Input: part model. Units: mm. Frame: model coordinates. A direction names the side the tool comes from. Round coordinates to 2 decimals unless told otherwise and drop trailing zeros. Loops run counter-clockwise (first coordinate to the right, second up) from the corner with the lowest first, then second, coordinate; pieces in that order, holes last. Notation, with made-up numbers: (-29.75, 12.25) -> (-18.75, 12.25) arc R29 ccw to (-18.75, 40.25) -> close; hole circle Ø5 at (-20, 30.25). An arc over 180 degrees is marked (long way). Answer in a Markdown table with one row per item. Add a question column.
Q1. Mould query, pull axis X, two halves, no side actions, for faces 5 (the face through (-103.049, 3, -23)), 6 (the face through (-40, 3, 61.274)), 7 (the face through (-148, 3, 116.519)), 8 (the face through (-128.449, 3, -23)). Classes: pulls with the +X half, pulls with the -X half, needs draft (parallel to the pull), parting line crosses it, or undercut.
Q2. Pin query (flat end, axial travel): pin 1 (1 mm diameter, centred on x = 1.5, y = 3, fed in from +Z); pin 2 (3.5 mm diameter, centred on y = 2, z = 73.5, fed in from +X); pin 3 (1.4 mm diameter, centred on x = 68.5, y = 4.5, fed in from -Z). Return the tip coordinate at first contact, or that it passes through.
Q3. Ray query, L1, parallel to X at y = 2.75, z = -17; L2, parallel to X at y = 5.5, z = 25; L3, parallel to X at y = 0.5, z = 34.5. Return the intervals inside material, ascending. Write a range as from..to.
Q4. Section B-B, the plane x = 21.5. Output: boundary loops of the cut face in (y, z), and give its area (3 significant figures).
Q5. Section C-C, the plane y = 4.5. Give the number of separate pieces and of enclosed holes in the cut face, and give its area (3 significant figures).
Q6. Reachability of faces 1 (the face through (49, 3, 19.999)), 2 (the face through (-128.449, 3, 120)), 3 (the face through (-103.049, 3, 120)), 4 (the face through (78, 3, 35.874)) from +Z, -Z, +X, -X, +Y, -Y: full face, straight path, thin tool, end or side. Return the list, or none.
Q7. Section A-A, the plane x = 50. Output: boundary loops of the cut face in (y, z), and give its area (3 significant figures).
```python
from build123d import *

# Parameters (mm, degrees)
SKETCH1_R           = 1.5875
SKETCH1_W           = 6.35
SKETCH1_H           = 25.4
BOSS_EXTRUDE1_DEPTH = 6.35


with BuildPart() as part:
    # Sketch1 → Boss-Extrude1 (new body)
    with BuildSketch(Plane(origin=(0, 0, 0), x_dir=(1, 0, 0), z_dir=(0, 1, 0))):
        Polygon((-153.849110766, 19.370876928), (-153.849110766, -116.519123072), (-142.673040444, -116.519123072), (-142.673040444, -113.344123072), (-144.425640444, -113.344123072), (-144.425640444, -110.804123072), (-142.673040444, -110.804123072), (-142.673040444, -109.534123072), (-139.625181088, -109.534123072), (-139.625181088, -110.804123072), (-137.872581088, -110.804123072), (-137.872581088, -113.344123072), (-139.625181088, -113.344123072), (-139.625181088, -116.519123072), (-128.449110766, -116.519123072), (-128.449110766, -122.869123072), (-103.049110766, -122.869123072), (-103.049110766, -116.519123072), (-91.873040444, -116.519123072), (-91.873040444, -113.344123072), (-93.625640444, -113.344123072), (-93.625640444, -110.804123072), (-91.873040444, -110.804123072), (-91.873040444, -109.534123072), (-88.825181088, -109.534123072), (-88.825181088, -110.804123072), (-87.072581088, -110.804123072), (-87.072581088, -113.344123072), (-88.825181088, -113.344123072), (-88.825181088, -116.519123072), (-77.649110766, -116.519123072), (74.750889234, -116.519123072), (81.100889234, -116.519123072), (81.100889234, -86.674123072), (74.750889234, -86.674123072), (74.750889234, -75.49805275), (71.575889234, -75.49805275), (71.575889234, -77.25065275), (69.035889234, -77.25065275), (69.035889234, -75.49805275), (67.765889234, -75.49805275), (67.765889234, -72.450193394), (69.035889234, -72.450193394), (69.035889234, -70.697593394), (71.575889234, -70.697593394), (71.575889234, -72.450193394), (74.750889234, -72.450193394), (74.750889234, -61.274123072), (81.100889234, -61.274123072), (81.100889234, -35.874123072), (74.750889234, -35.874123072), (74.750889234, -24.69805275), (71.575889234, -24.69805275), (71.575889234, -26.45065275), (69.035889234, -26.45065275), (69.035889234, -24.69805275), (67.765889234, -24.69805275), (67.765889234, -21.650193394), (69.035889234, -21.650193394), (69.035889234, -19.897593394), (71.575889234, -19.897593394), (71.575889234, -21.650193394), (74.750889234, -21.650193394), (74.750889234, -10.474123072), (81.100889234, -10.474123072), (81.100889234, 19.370876928), (74.750889234, 19.370876928), (-77.649110766, 19.370876928), (-88.825181088, 19.370876928), (-88.825181088, 16.195876928), (-87.072581088, 16.195876928), (-87.072581088, 13.655876928), (-88.825181088, 13.655876928), (-88.825181088, 12.385876928), (-91.873040444, 12.385876928), (-91.873040444, 13.655876928), (-93.625640444, 13.655876928), (-93.625640444, 16.195876928), (-91.873040444, 16.195876928), (-91.873040444, 19.370876928), (-103.049110766, 19.370876928), (-103.049110766, 25.720876928), (-128.449110766, 25.720876928), (-128.449110766, 19.370876928), (-139.625181088, 19.370876928), (-139.625181088, 16.195876928), (-137.872581088, 16.195876928), (-137.872581088, 13.655876928), (-139.625181088, 13.655876928), (-139.625181088, 12.385876928), (-142.673040444, 12.385876928), (-142.673040444, 13.655876928), (-144.425640444, 13.655876928), (-144.425640444, 16.195876928), (-142.673040444, 16.195876928), (-142.673040444, 19.370876928), align=None)
        with Locations(Location((-39.549110766, 2.225876928, 0), (0, 0, 270))):
            Circle(SKETCH1_R, mode=Mode.SUBTRACT)
        with Locations(Location((-39.549110766, -48.574123072, 0), (0, 0, 270))):
            Circle(SKETCH1_R, mode=Mode.SUBTRACT)
        with Locations(Location((-39.549110766, -99.374123072, 0), (0, 0, 270))):
            Circle(SKETCH1_R, mode=Mode.SUBTRACT)
        with Locations(Location((77.925889234, 2.225876928, 0), (0, 0, 270))):
            Circle(SKETCH1_R, mode=Mode.SUBTRACT)
        with Locations(Location((77.925889234, -48.574123072, 0), (0, 0, 270))):
            Circle(SKETCH1_R, mode=Mode.SUBTRACT)
        with Locations(Location((77.925889234, -99.374123072, 0), (0, 0, 270))):
            Circle(SKETCH1_R, mode=Mode.SUBTRACT)
        with Locations(Location((62.050889234, -80.324123072, 0), (0, 0, 270))):
            Circle(SKETCH1_R, mode=Mode.SUBTRACT)
        with Locations(Location((62.050889234, -16.824123072, 0), (0, 0, 270))):
            Circle(SKETCH1_R, mode=Mode.SUBTRACT)
        with Locations((-39.549110766, -23.174123072)):
            Rectangle(SKETCH1_W, SKETCH1_H, mode=Mode.SUBTRACT)
        with Locations((-39.549110766, -73.974123072)):
            Rectangle(SKETCH1_W, SKETCH1_H, mode=Mode.SUBTRACT)
        Polygon((49.350889234, -77.149123072), (43.000889234, -77.149123072), (43.000889234, -83.499123072), (55.700889234, -83.499123072), (55.700889234, -77.149123072), align=None, mode=Mode.SUBTRACT)
        Polygon((49.350889234, -19.999123072), (43.000889234, -19.999123072), (43.000889234, -13.649123072), (55.700889234, -13.649123072), (55.700889234, -19.999123072), align=None, mode=Mode.SUBTRACT)
    extrude(amount=BOSS_EXTRUDE1_DEPTH)


solid = part.part
```
Answer block:
| question | item | result |
|---|---|---|
| 1 | face 5 | pulls with the +X half |
| 1 | face 6 | undercut |
| 1 | face 7 | needs draft |
| 1 | face 8 | pulls with the -X half |
| 2 | pin 1 | z = 116.52 |
| 2 | pin 2 | x = 74.75 |
| 2 | pin 3 | z = -19.37 |
| 3 | L1 | -153.85..-142.67, -139.63..-91.87, -88.83..81.1 |
| 3 | L2 | -153.85..-42.72, -36.37..69.04, 71.58..74.75 |
| 3 | L3 | -153.85..-42.72, -36.37..74.75 |
| 4 | outline | (0, -19.37) -> (6.35, -19.37) -> (6.35, 116.52) -> (0, 116.52) -> close |
| 4 | area | 863 mm^2 |
| 5 | separate pieces | 1 |
| 5 | enclosed holes | 12 |
| 5 | area | 31,200 mm^2 |
| 6 | face 1 | +Y, -Y |
| 6 | face 2 | +Z, -X, +Y, -Y |
| 6 | face 3 | +Z, +X, +Y, -Y |
| 6 | face 4 | +X, +Y, -Y |
| 7 | outline | (0, -19.37) -> (6.35, -19.37) -> (6.35, 13.65) -> (0, 13.65) -> close; (0, 20) -> (6.35, 20) -> (6.35, 77.15) -> (0, 77.15) -> close; (0, 83.5) -> (6.35, 83.5) -> (6.35, 116.52) -> (0, 116.52) -> close |
| 7 | area | 782 mm^2 |
